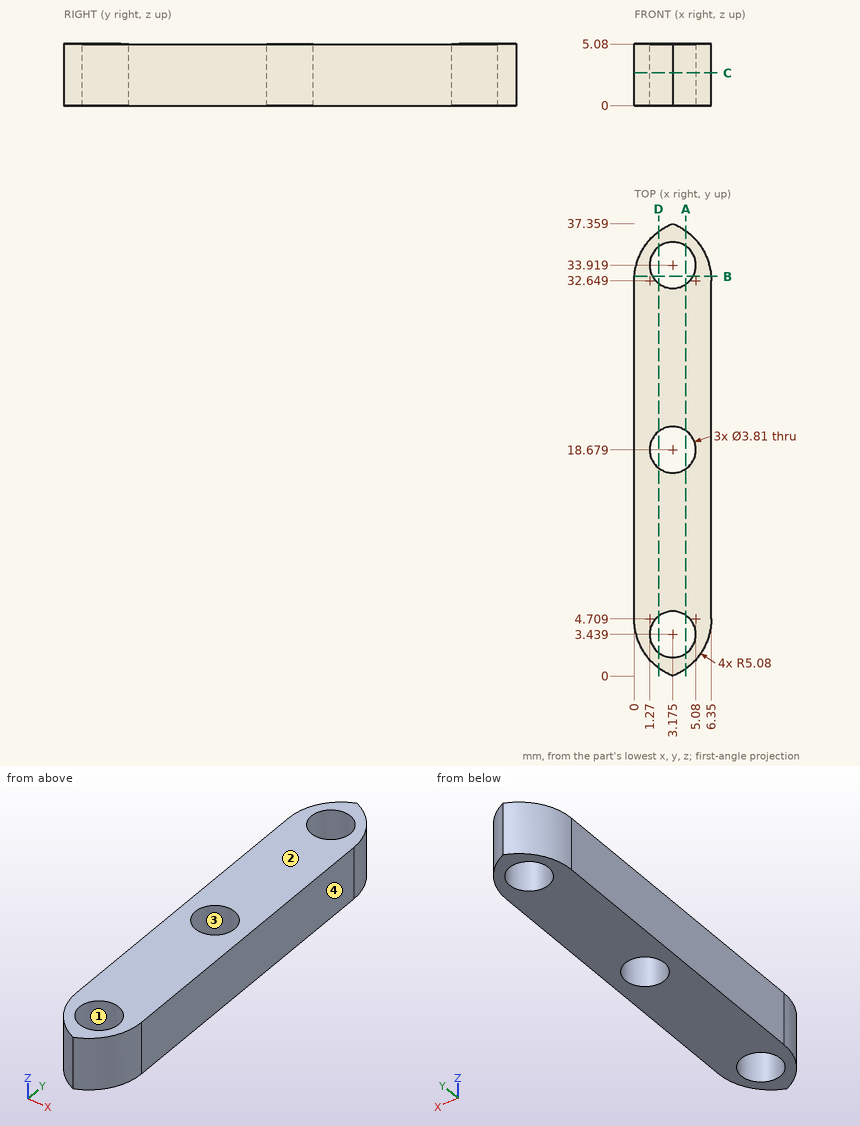
Study the drawing (mm; zero at the part's minimum x, y, z) and answer. Round coordinates to 2 decimals unless told otherwise and drop trailing zeros. Write each loop counter-clockwise with the first axis right and the second up, starting at its lowest first coordinate (ties: lowest second). Pieces come first, ordered by that corner, then holes.
1) A cutting plane is placed at C-C on z = 2.7. Give the number of separate pieces and of enclosed holes in the cut face.
2) A cutting plane is placed at D-D on x = 2. Determine the outline of the cut face in (y, z).
3) A cutting plane is placed at A-A on x = 4.25. Determine the outline of the cut face in (y, z) (1 decimal).
4) Determine the mould class of the marked faces 1, 2, 3 and 4 for opening direction X: pulls with the +X half, pulls with the -X half, needs draft (parallel to the pull), parting line crosses it, or undercut.
5) Flat-ended cylindrical pins translate along their axes: P1, Ø3, axis at x = 3.5, y = 10.5, coming from the -Z side; P2, Ø1, axis at x = 4, z = 1.5, coming from the -Y side (1 decimal). Find the tip coordinate at first contact, or state that the pin passes through.
6) A cutting plane is placed at B-B on y = 33. Determine the outline of the cut face in (x, z).
7) Consider probe 1 along Y at (x, z) = (2.25, 1) (1 decimal); probe 2 along Y at (x, z) = (4.5, 3.2); probe 3 along X at (y, z) = (35, 1.8) (1 decimal). Determine where each line is inside the solid, lowest interval first.
Entries:
1. separate pieces: 1
1. enclosed holes: 3
2. outline: (0.67, 0) - (1.94, 0) - (1.94, 5.08) - (0.67, 5.08) - close; (4.94, 0) - (17.18, 0) - (17.18, 5.08) - (4.94, 5.08) - close; (20.18, 0) - (32.42, 0) - (32.42, 5.08) - (20.18, 5.08) - close; (35.42, 0) - (36.69, 0) - (36.69, 5.08) - (35.42, 5.08) - close
3. outline: (0.6, 0) - (1.9, 0) - (1.9, 5.1) - (0.6, 5.1) - close; (5, 0) - (17.1, 0) - (17.1, 5.1) - (5, 5.1) - close; (20.3, 0) - (32.3, 0) - (32.3, 5.1) - (20.3, 5.1) - close; (35.5, 0) - (36.8, 0) - (36.8, 5.1) - (35.5, 5.1) - close
4. face 1: undercut
4. face 2: needs draft
4. face 3: undercut
4. face 4: pulls with the +X half
5. P1: stops at z = 0
5. P2: stops at y = 0.1
6. outline: (0.01, 0) - (1.51, 0) - (1.51, 5.08) - (0.01, 5.08) - close; (4.84, 0) - (6.34, 0) - (6.34, 5.08) - (4.84, 5.08) - close
7. probe 1: y = 0.5 to 1.8, 5.1 to 17, 20.3 to 32.3, 35.6 to 36.9
7. probe 2: y = 0.79 to 2.07, 4.81 to 17.31, 20.05 to 32.55, 35.29 to 36.57
7. probe 3: x = 0.6 to 1.6, 4.7 to 5.8
